For this review, take the finished solid that the model builds, in its own axes (mm). Face numbers are marked on the shaded views. A direction names the side the tool comes from. Round coordinates to 2 decimals unless told otherwise and drop trailing zeros. Write each loop counter-clockwise with the first axis right and the second up, starting at its lowest first coordinate (ties: lowest second). Pieces come first, ordered by that corner, then holes. Notation, with made-up numbers: (-40, 86.25) -> (6, 86.25) arc R20 ccw to (6, 97.25) -> close; hole circle Ø10 at (78.25, 53.25). An arc over 180 degrees is marked (long way). Answer as CSV lines item,"result". Start each with the question number.
Item 1: Take a section at A-A on y = 0. Give the boundary of the cut face in (x, z).
Item 2: Take a section at D-D on y = 11. Give the boundary of the cut face in (x, z).
Item 3: Wall thickness on probe 1 along Z at (x, y) = (-10, -2); probe 2 along X at (y, z) = (-4, 14); probe 3 along X at (y, z) = (16, 50): over which ranges is each line inside the solid? List them lowest first. Write a range as from..to.
Item 4: For pin 1 Ø2 at (y, z) = (-14, 56) entering from +X; pin 2 Ø6 at (x, y) = (10.5, 0.5) entering from +Z; pin 3 Ø3 at (x, y) = (4, -10.5) entering from +Z, all flat-tipped, find the tip position at first contact; note any pin that passes through.
Item 5: Mouldability with a two-part tool opening along Z and no side actions: class the marked faces 1, 2 and 3 as +Z half, -Z half, draft (parallel to the pull), parting line (faces both ways), or undercut.
Item 6: Take a section at C-C on x = 1. Give the boundary of the cut face in (y, z).
Item 7: Take a section at B-B on z = 14.5. Give the boundary of the cut face in (x, y), then the cut area to 3 significant figures.
Item 8: Machinability: for the marked faces 4, 5, 6, 7 and 8, which of the approach directions +Z, -Z, +X, -X, +Y, -Y give a long, thin tool a straight path to every point of the face, cutting with its end or side? Answer none if there is none.
```python
from build123d import *

# Parameters (mm, degrees)
F1_DEPTH = 22.352
F2_R     = 7.432134
F3_DEPTH = 25.4


with BuildPart() as f1:
    # F0 (on Top) → F1 (new body)
    with BuildSketch(Plane.XY):
        Polygon((13.858515, -8.001217), (13.858515, 8.001217), (0, 16.002435), (-13.858515, 8.001217), (-13.858515, -8.001217), (0, -16.002435), align=None)
    extrude(amount=F1_DEPTH)

    # F2 (on face) → F3 (join)
    with BuildSketch(Plane.XY.offset(22.352)):
        Circle(F2_R)
    extrude(amount=F3_DEPTH)

    # F4 (on face) → F5 (revolve)
    with BuildSketch(Plane.XY.offset(47.752)):
        with BuildLine():
            Line((7.432134, 0), (20.542542, 0))
            ThreePointArc((20.542542, 0), (0, 20.542542), (-20.542542, 0))
            Line((-20.542542, 0), (-7.432134, 0))
            ThreePointArc((-7.432134, 0), (0, 7.432134), (7.432134, 0))
        make_face()
        with BuildLine():
            Line((-7.432134, 0), (7.432134, 0))
            ThreePointArc((7.432134, 0), (0, 7.432134), (-7.432134, 0))
        make_face()
    revolve(axis=Axis((0, 0, 47.752), (-1, 0, 0)))


solid = f1.part
```
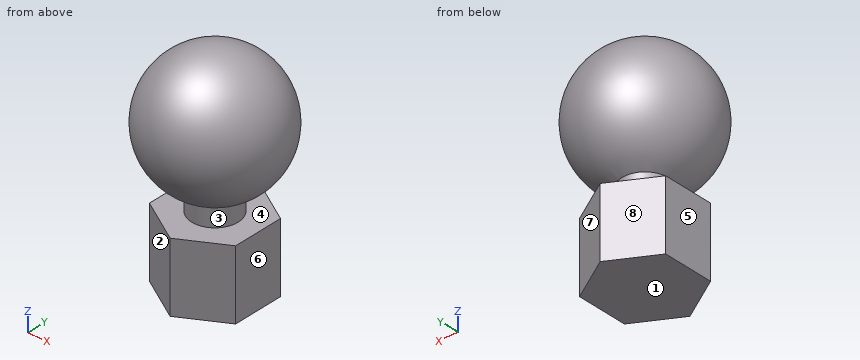
Output values:
1,outline,"(-13.86, 0) -> (13.86, 0) -> (13.86, 22.35) -> (7.43, 22.35) -> (7.43, 28.6) arc R20.54 ccw (long way) to (-7.43, 28.6) -> (-7.43, 22.35) -> (-13.86, 22.35) -> close"
2,outline,"circle Ø34.7 at (0, 47.75); (-8.66, 0) -> (8.66, 0) -> (8.66, 22.35) -> (-8.66, 22.35) -> close"
3,probe 1,"z = 0..22.35, 29.92..65.58"
3,probe 2,"x = -13.86..13.86"
3,probe 3,"x = -12.69..12.69"
4,pin 1,"stops at x = 13.76"
4,pin 2,"stops at z = 66.87"
4,pin 3,"stops at z = 65.84"
5,face 1,"-Z half"
5,face 2,"draft"
5,face 3,"undercut"
6,outline,"(-15.43, 0) -> (15.43, 0) -> (15.43, 22.35) -> (7.36, 22.35) -> (7.36, 28.6) arc R20.52 ccw (long way) to (-7.36, 28.6) -> (-7.36, 22.35) -> (-15.43, 22.35) -> close"
7,outline,"(-13.86, -8) -> (0, -16) -> (13.86, -8) -> (13.86, 8) -> (0, 16) -> (-13.86, 8) -> close"
7,area,"665 mm^2"
8,face 4,"none"
8,face 5,"-Z, -X, +Y, -Y"
8,face 6,"-Z, +X, +Y, -Y"
8,face 7,"-Z, +X, +Y"
8,face 8,"-Z, -X, +Y"
